Can you work these out from the drawing? Everything is in mm from the part's minimum corner. A direction names the side the tool comes from. Coordinates: 2 decimals unless noted, no trailing zeros. Order: outer loops, then holes, each group sorted by start corner. A loop starts at its lowest first (then second) coordinate and runs counter-clockwise, first axis right, second up. Notation, with made-up numbers: M 77.25,-4 L 85.25,-4 A19 cw 85.25,1 Z; hole C -4,31 d6. An arc over 180 degrees is marked long. Answer as CSV lines item,"result". Start each with the question number.
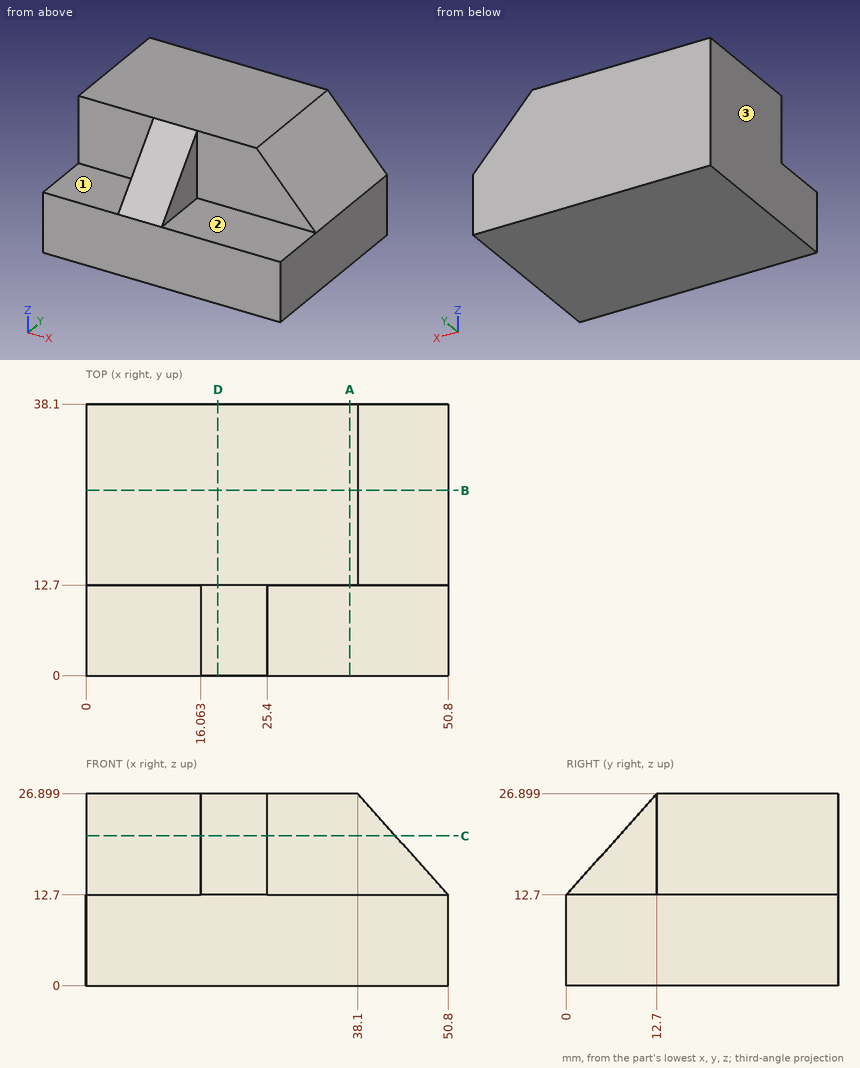
1) Suppose I cut it at C-C on z = 21. Please give me the cut outline in (x, y).
2) Which directions (+Z, -Z, +X, -X, +Y, -Y) give clear straight access to the entire face, cutting with the end or side of a thin tool? Please do the marked faces 1, 2 and 3.
3) Suppose I cut it at D-D on x = 18.5. Please give me the cut outline in (y, z), plus the area to 3 significant figures.
4) I need wall thicknesses on line 1 (Z direction, x = 4, y = 4); line 2 (Y direction, x = 27, z = 12.75); line 3 (X direction, y = 11.5, z = 23.5). Which ranges of each line are inside material? Lowest first, please. Write a range as [from, to].
5) Suppose I cut it at A-A on x = 37. Please give me the cut outline in (y, z).
6) Suppose I cut it at B-B on y = 26. Please give me the cut outline in (x, z), plus the area to 3 significant figures.
7) Will these pins go through, and if not, where does the flat tip stop? pin 1 Ø4 at (x, y) = (39.5, 5.5) entering from +Z; pin 2 Ø4.5 at (x, z) = (43, 22) entering from -Y; pin 3 Ø6.5 at (y, z) = (9, 23) entering from +X.
Output:
1,outline,"M 0,12.7 L 16.06,12.7 L 16.06,7.42 L 25.4,7.42 L 25.4,12.7 L 43.38,12.7 L 43.38,38.1 L 0,38.1 Z"
2,face 1,"+Z, -X, -Y"
2,face 2,"+Z, +X, -Y"
2,face 3,"+Z, -Z, -X, +Y, -Y"
3,outline,"M 0,0 L 38.1,0 L 38.1,26.9 L 12.7,26.9 L 0,12.7 Z"
3,area,"935 mm²"
4,line 1,"[0, 12.7]"
4,line 2,"[12.7, 38.1]"
4,line 3,"[16.06, 25.4]"
5,outline,"M 0,0 L 38.1,0 L 38.1,26.9 L 12.7,26.9 L 12.7,12.7 L 0,12.7 Z"
6,outline,"M 0,0 L 50.8,0 L 50.8,12.7 L 38.1,26.9 L 0,26.9 Z"
6,area,"1,280 mm²"
7,pin 1,"z = 12.7"
7,pin 2,"y = 12.7"
7,pin 3,"x = 25.4"
